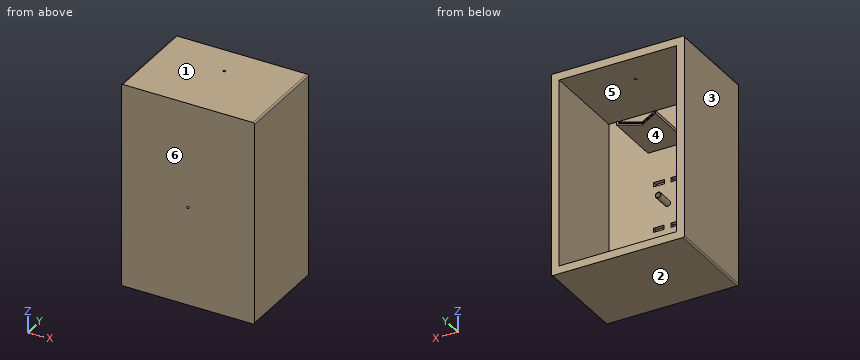
Autodesk Inventor part; units mm, degrees
ref_plane "YZ Plane" through (0, 0, 0) normal (1, 0, 0) x (0, 1, 0)
ref_plane "XZ Plane" through (0, 0, 0) normal (0, 1, 0) x (-1, 0, 0)
ref_plane "XY Plane" through (0, 0, 0) normal (0, 0, 1) x (1, 0, 0)
sketch "Boceto1" plane through (0, 0, 0) normal (0, 1, 0) x (-1, 0, 0)
  line L0 (-85, -130) -> (85, -130)
  line L1 (85, -130) -> (85, 130)
  line L2 (85, 130) -> (-85, 130)
  line L3 (-85, 130) -> (-85, -130)
  line L4 (-85, -130) -> (85, 130) construction
  line L5 (85, -130) -> (-85, 130) construction
  line L6 (75, 120) -> (75, -120)
  line L7 (75, -120) -> (-75, -120)
  line L8 (-75, -120) -> (-75, 120)
  line L9 (-75, 120) -> (75, 120)
  point P0 (0, 0)
  point P1 (0, -120)
  point P2 (0, 120)
  point P3 (0, 0)
  dimension "d0" = 170
  dimension "d1" = 260
  dimension "d10" = 10
extrude "Extrusión1" add sketch "Boceto1" along normal blind 121
extrude "Extrusión3" add sketch "Boceto1" along normal blind 10 contours L6 L7 L8 L9
sketch "Boceto4" plane through (0, 10, 0) normal (0, 1, 0) x (1, 0, 0)
  circle A0 centre (0, 4.19) radius 3.75
  line L0 (85, 130) -> (-85, 130)
  circle A1 centre (0, 4.19) radius 3.35
  circle A2 centre (0, 4.19) radius 1.5
  line L1 (-85, -130) -> (85, -130)
  line L2 (75, -120) -> (-75, -120) construction
  line L3 (0, -120) -> (0, -70) construction
  point P0 (0, 0)
  dimension "d15" = 7.5
  dimension "d17" = 0.4
  dimension "d20" = 3
  dimension "d23" = 134.19
  dimension "d36" = 50
extrude "Extrusión4" add sketch "Boceto4" along normal blind 21 contours A0
extrude "Extrusión5" cut sketch "Boceto4" against normal blind 10 contours A2
sketch "Boceto7" plane through (0, 10, 0) normal (0, 1, 0) x (1, 0, 0)
  circle A0 centre (0, 4.19) radius 1.5 construction
  line L0 (0, 4.19) -> (-17.5, 4.19) construction
  circle A1 centre (0, 4.19) radius 1.5 construction
  line L1 (0, 4.19) -> (0, -27.68) construction
  line L2 (75, -120) -> (-75, -120) construction
  line L3 (0, -120) -> (0, -70) construction
  line L4 (0, -70) -> (-19.0745, -70) construction
  line L5 (25, -68) -> (-25, -68)
  line L6 (-25, -68) -> (-25, -72)
  line L7 (-25, -72) -> (25, -72)
  line L8 (25, -72) -> (25, -68)
  line L9 (25, -68) -> (-25, -72) construction
  line L10 (-25, -68) -> (25, -72) construction
  line L11 (-23.5, -70.5) -> (-23.5, -69.5)
  line L12 (-23.5, -69.5) -> (23.5, -69.5)
  line L13 (23.5, -69.5) -> (23.5, -70.5)
  line L14 (23.5, -70.5) -> (-23.5, -70.5)
  line L15 (-4.25, -22.43) -> (-17.75, -22.43)
  line L16 (-17.75, -22.43) -> (-17.75, -27.93)
  line L17 (-17.75, -27.93) -> (-4.25, -27.93)
  line L18 (-4.25, -27.93) -> (-4.25, -22.43)
  line L19 (17.75, -22.43) -> (4.25, -22.43)
  line L20 (4.25, -22.43) -> (4.25, -27.93)
  line L21 (4.25, -27.93) -> (17.75, -27.93)
  line L22 (17.75, -27.93) -> (17.75, -22.43)
  line L23 (-4.25, 36.31) -> (-17.75, 36.31)
  line L24 (-17.75, 36.31) -> (-17.75, 30.81)
  line L25 (-17.75, 30.81) -> (-4.25, 30.81)
  line L26 (-4.25, 30.81) -> (-4.25, 36.31)
  line L27 (18.25, 36.31) -> (4.75, 36.31)
  line L28 (4.75, 36.31) -> (4.75, 30.81)
  line L29 (4.75, 30.81) -> (18.25, 30.81)
  line L30 (18.25, 30.81) -> (18.25, 36.31)
  point P0 (0, 0)
  dimension "d43" = 31.87
  dimension "d44" = 50
  dimension "d45" = 50
  dimension "d46" = 4
  dimension "d47" = 1.5
  dimension "d100" = 13.5
  dimension "d101" = 5.5
  dimension "d102" = 13.5
  dimension "d103" = 5.5
  dimension "d104" = 13.5
  dimension "d105" = 5.5
  dimension "d106" = 13.5
  dimension "d107" = 5.5
sketch "Boceto8" plane through (75, 121, 120) normal (0, 0, -1) x (-1, 0, 0)
  line L0 (0, -111) -> (150, -111) construction
  line L1 (75, -111) -> (75, -11) construction
  circle A0 centre (75, -40) radius 5
  circle A1 centre (75, -40) radius 1.5
  point P0 (75, -121)
  dimension "d37" = 100
  dimension "d38" = 10
  dimension "d75" = 3
extrude "Extrusión9" add sketch "Boceto7" along normal blind 71 contours L8 L7 L6 L5
sketch "Boceto9" plane through (-25, 10, 72) normal (0, 0, 1) x (1, 0, 0)
  line L0 (0, 71) -> (25, 56.5662)
  line L1 (0, 71) -> (57.416, 71) construction
  line L2 (50, 71) -> (25, 56.5662)
  line L3 (50, 71) -> (104.7106, 71) construction
  arc A0 (48.8838, 70.3556) -> (1.1162, 70.3556) centre (25, 56.5662) ccw
  line L4 (0, 71) -> (1.5, 71)
  line L5 (0, 71) -> (50, 71)
  line L6 (50, 71) -> (48.5, 71)
  point P0 (25, -10)
extrude "Extrusión11" add sketch "Boceto9" against normal blind 4 contours A0 L5 L2 L0 | A0 L5
extrude "Extrusión12" cut sketch "Boceto9" against normal blind 4 contours A0 L5 L2 L0 | A0 L5
extrude "Extrusión13" cut sketch "Boceto9" against normal blind 4 contours L4 A0 L0
extrude "Extrusión14" cut sketch "Boceto9" against normal blind 4 contours L5 L2 A0
extrude "Extrusión15" [suppressed]
extrude "Extrusión16" [suppressed]
fillet "Empalme1" radius 2 4 edges at (85, 60.5, 130) (-85, 60.5, 130) (85, 60.5, -130) (-85, 60.5, -130)
extrude "Extrusión17" cut sketch "Boceto8" against normal through all contours A1
extrude "Extrusión20" cut sketch "Boceto7" against normal blind 5 contours L18 L17 L16 L15 | L22 L21 L20 L19 | L26 L25 L24 L23 | L30 L29 L28 L27
properties part number "BoxDark"
Here's how the part is built. I have some questions about the finished solid (model axes, mm). Face numbers are marked on the shaded views. A direction names the side the tool comes from. Round coordinates to 2 decimals unless told otherwise and drop trailing zeros. Order: outer loops, then holes, each group sorted by start corner. A loop starts at its lowest first (then second) coordinate and runs counter-clockwise, first axis right, second up. Notation, with made-up numbers: (-19, 74) -> (30, 74) arc R19 ccw to (30, 79) -> close; hole circle Ø5 at (-38.75, 12.5). An arc over 180 degrees is marked (long way). Use a Markdown table: item, result. Add a question column.
(1) Suppose I cut it at A-A, the plane y = 60. Please give me the cut outline in (x, z), and give its area (3 significant figures).
(2) For pin 1 Ø6 at (x, z) = (11, 25.5) entering from +Y; pin 2 Ø1.6 at (x, z) = (-10.5, 26) entering from +Y, each with a flat end and sliding along its axis, tell me the tip position at first contact or that it passes through.
(3) Suppose I cut it at B-B, the plane z = 103. Please give me the cut outline in (x, y), and give its area (3 significant figures).
(4) If we mould it in two halves opening along Z, with no side actions, what happens to the marked faces 1, 2, 3 and 4? For each: released by +Z, released by -Z, zero draft, split by the parting line, or undercut.
(5) Suppose I cut it at D-D, the plane x = -11.5. Please give me the cut outline in (y, z), and give its area (3 significant figures).
(6) I need wall thicknesses on line 1 along Z through (x, y) = (0, 20.75); line 2 along X through (y, z) = (20.25, -4.19); line 3 along X through (y, z) = (65.5, -1.5). Which ranges of each line are inside material? Lowest first, please.
(7) Suppose I cut it at C-C, the plane x = -50. Please give me the cut outline in (y, z), and give its area (3 significant figures).
(8) For the marked faces 5 and 6, which set-ups out of +Z, -Z, +X, -X, +Y, -Y let a thin tool reach every point of the face, with its end or its side?
Verdict:
| question | item | result |
|---|---|---|
| 1 | outline | (-85, -128) arc R2 ccw to (-83, -130) -> (83, -130) arc R2 ccw to (85, -128) -> (85, 128) arc R2 ccw to (83, 130) -> (-83, 130) arc R2 ccw to (-85, 128) -> close; (-25, 68) -> (25, 68) -> (25, 72) -> (-25, 72) -> close; hole (-75, -120) -> (75, -120) -> (75, 120) -> (-75, 120) -> close; hole (-23.5, 69.5) -> (23.5, 69.5) -> (23.5, 70.5) -> (-23.5, 70.5) -> close |
| 1 | area | 8,350 mm2 |
| 2 | pin 1 | y = 10 |
| 2 | pin 2 | y = 5 |
| 3 | outline | (-85, 0) -> (85, 0) -> (85, 121) -> (75, 121) -> (75, 10) -> (-75, 10) -> (-75, 121) -> (-85, 121) -> close |
| 3 | area | 3,920 mm2 |
| 4 | face 1 | released by +Z |
| 4 | face 2 | released by -Z |
| 4 | face 3 | zero draft |
| 4 | face 4 | undercut |
| 5 | outline | (0, -130) -> (121, -130) -> (121, -120) -> (10, -120) -> (10, -36.31) -> (5, -36.31) -> (5, -30.81) -> (10, -30.81) -> (10, 22.43) -> (5, 22.43) -> (5, 27.93) -> (10, 27.93) -> (10, 68) -> (73.21, 68) -> (73.21, 69.5) -> (10, 69.5) -> (10, 70.5) -> (73.21, 70.5) -> (73.21, 72) -> (10, 72) -> (10, 120) -> (121, 120) -> (121, 130) -> (0, 130) -> close |
| 5 | area | 4,950 mm2 |
| 6 | line 1 | -130 to -120, -7.94 to -7.54, -0.84 to -0.44, 68 to 69.5, 70.5 to 72, 120 to 130 |
| 6 | line 2 | -85 to -75, -3.75 to -3.35, 3.35 to 3.75, 75 to 85 |
| 6 | line 3 | -85 to -75, 75 to 85 |
| 7 | outline | (0, -130) -> (121, -130) -> (121, -120) -> (10, -120) -> (10, 120) -> (121, 120) -> (121, 130) -> (0, 130) -> close |
| 7 | area | 4,820 mm2 |
| 8 | face 5 | +Y |
| 8 | face 6 | +Z, -Z, +X, -X, -Y |
